For this review, take the finished solid that the model builds, in its own axes (mm). Round coordinates to 2 decimals unless told otherwise and drop trailing zeros. Loops run counter-clockwise (first coordinate to the right, second up) from the corner with the lowest first, then second, coordinate; pieces in that order, holes last. Notation, with made-up numbers: (43.5, -26.75) -> (80.5, -26.75) arc R18 cw to (80.5, -0.75) -> close; hole circle Ø11 at (84, 13). An arc over 180 degrees is marked (long way). One line per question, with ' | ' between items. Start each with the question number.
1. Draft analysis for pull direction Y (two halves, no side actions). For faces 1 (the face through (97, 79, 0)), 2 (the face through (46.24, 97.88, 1.48)), state which applies: pulls with the +Y half, pulls with the -Y half, needs draft (parallel to the pull), parting line crosses it, or undercut.
2. Wall thickness on line 1 along Y through (x, z) = (64.5, 2.1); line 2 along Y through (x, z) = (52.5, 1.65); line 3 along Y through (x, z) = (45.5, 2.45): over which ranges is each line inside the solid? List them lowest first.
3. Consider section A-A (y = 139.5). Write out the cut boundary in (x, z).
4. For pin 1 Ø5.5 at (x, y) = (95.5, 73.8) entering from +Z, flat-tipped, find the tip position at first contact; note if it passes through.
5. Consider section B-B (z = 1.55). Count the separate pieces of the cut face and the enclosed holes in it, and give its area (3 significant figures).
6. Consider section C-C (x = 27.5). Write out the cut boundary in (y, z), and give its area (3 significant figures).
```python
from build123d import *

# Parameters (mm, degrees)
MODEL_R                         = 3.59
MODEL_R_2                       = 2.55
MODEL_R_3                       = 1.7
MODEL_R_4                       = 2.7
AUFSATZ_LINEAR_AUSTRAGEN1_DEPTH = 3


with BuildPart() as part:
    # Model → Aufsatz-Linear austragen1 (new body)
    with BuildSketch(Plane.XY):
        with BuildLine():
            Line((157, 155), (47.6787101, 155))
            ThreePointArc((47.6787101, 155), (42.610842111, 153.620714242), (38.94098175, 149.86334281))
            Line((38.94098175, 149.86334281), (1.26227165, 82.167861266))
            ThreePointArc((1.26227165, 82.167861266), (0.32071068, 79.816760135), (0, 77.304518457))
            Line((0, 77.304518457), (0, 10))
            ThreePointArc((0, 10), (2.928932188, 2.928932188), (10, 0))
            Line((10, 0), (150, 0))
            ThreePointArc((150, 0), (157.071067812, 2.928932188), (160, 10))
            Line((160, 10), (160, 152))
            ThreePointArc((160, 152), (159.121320344, 154.121320344), (157, 155))
        make_face()
        with Locations((12.7, 12.7)):
            Circle(MODEL_R, mode=Mode.SUBTRACT)
        with Locations((47.7, 12.7)):
            Circle(MODEL_R, mode=Mode.SUBTRACT)
        with Locations((147.3, 12.7)):
            Circle(MODEL_R, mode=Mode.SUBTRACT)
        with Locations((47.7, 145)):
            Circle(MODEL_R, mode=Mode.SUBTRACT)
        with Locations((112.3, 145)):
            Circle(MODEL_R_2, mode=Mode.SUBTRACT)
        with Locations((52.5, 76.5)):
            Circle(MODEL_R_2, mode=Mode.SUBTRACT)
        with Locations((107.5, 76.5)):
            Circle(MODEL_R_2, mode=Mode.SUBTRACT)
        with Locations((64.5, 39)):
            Circle(MODEL_R_2, mode=Mode.SUBTRACT)
        with Locations((95.5, 39)):
            Circle(MODEL_R_2, mode=Mode.SUBTRACT)
        with Locations((64.5, 61.8)):
            Circle(MODEL_R_3, mode=Mode.SUBTRACT)
        with Locations((64.5, 73.8)):
            Circle(MODEL_R_3, mode=Mode.SUBTRACT)
        with Locations((64.5, 92.8)):
            Circle(MODEL_R_3, mode=Mode.SUBTRACT)
        with Locations((64.5, 104.8)):
            Circle(MODEL_R_3, mode=Mode.SUBTRACT)
        with Locations((95.5, 61.8)):
            Circle(MODEL_R_3, mode=Mode.SUBTRACT)
        with Locations((95.5, 73.8)):
            Circle(MODEL_R_3, mode=Mode.SUBTRACT)
        with Locations((95.5, 92.8)):
            Circle(MODEL_R_3, mode=Mode.SUBTRACT)
        with Locations((95.5, 104.8)):
            Circle(MODEL_R_3, mode=Mode.SUBTRACT)
        with Locations((56.38, 53.68)):
            Circle(MODEL_R_4, mode=Mode.SUBTRACT)
        with Locations((103.62, 53.68)):
            Circle(MODEL_R_4, mode=Mode.SUBTRACT)
        with Locations((103.62, 100.92)):
            Circle(MODEL_R_4, mode=Mode.SUBTRACT)
        with Locations((56.38, 100.92)):
            Circle(MODEL_R_4, mode=Mode.SUBTRACT)
        with Locations((70, 145)):
            Circle(MODEL_R_4, mode=Mode.SUBTRACT)
        with Locations((150, 145)):
            Circle(MODEL_R_4, mode=Mode.SUBTRACT)
        with Locations((150, 125)):
            Circle(MODEL_R_4, mode=Mode.SUBTRACT)
        with Locations((108.8, 139.5)):
            Circle(MODEL_R_2, mode=Mode.SUBTRACT)
        with Locations((80, 61.8)):
            Circle(MODEL_R_4, mode=Mode.SUBTRACT)
        with Locations((113.403724343, 95.203724343)):
            Circle(MODEL_R_4, mode=Mode.SUBTRACT)
        with Locations((80, 128.607448687)):
            Circle(MODEL_R_4, mode=Mode.SUBTRACT)
        with Locations((46.596275657, 95.203724343)):
            Circle(MODEL_R_4, mode=Mode.SUBTRACT)
        with Locations((90, 10)):
            Circle(MODEL_R_4, mode=Mode.SUBTRACT)
        with Locations((70, 10)):
            Circle(MODEL_R_4, mode=Mode.SUBTRACT)
        with Locations((69.999999708, 125.000000186)):
            Circle(MODEL_R_4, mode=Mode.SUBTRACT)
        with BuildLine():
            Line((68.75, 89.3), (68.75, 77.3))
            ThreePointArc((68.75, 77.3), (80, 66.05), (91.25, 77.3))
            Line((91.25, 77.3), (91.25, 89.3))
            ThreePointArc((91.25, 89.3), (80, 100.55), (68.75, 89.3))
        make_face(mode=Mode.SUBTRACT)
        with BuildLine():
            Line((130, 147.7), (125, 147.7))
            ThreePointArc((125, 147.7), (122.3, 145), (125, 142.3))
            Line((125, 142.3), (130, 142.3))
            ThreePointArc((130, 142.3), (132.7, 145), (130, 147.7))
        make_face(mode=Mode.SUBTRACT)
        with BuildLine():
            Line((129.999999456, 127.699999985), (124.999999456, 127.699999985))
            ThreePointArc((124.999999456, 127.699999985), (122.299999456, 124.999999985), (124.999999456, 122.299999985))
            Line((124.999999456, 122.299999985), (129.999999456, 122.299999985))
            ThreePointArc((129.999999456, 122.299999985), (132.699999456, 124.999999985), (129.999999456, 127.699999985))
        make_face(mode=Mode.SUBTRACT)
        with BuildLine():
            Line((99.999999456, 127.699999985), (89.999999456, 127.699999985))
            ThreePointArc((89.999999456, 127.699999985), (87.299999456, 124.999999985), (89.999999456, 122.299999985))
            Line((89.999999456, 122.299999985), (99.999999456, 122.299999985))
            ThreePointArc((99.999999456, 122.299999985), (102.699999456, 124.999999985), (99.999999456, 127.699999985))
        make_face(mode=Mode.SUBTRACT)
        with BuildLine():
            Line((99.999999587, 147.700000259), (89.999999587, 147.700000259))
            ThreePointArc((89.999999587, 147.700000259), (87.299999587, 145.000000259), (89.999999587, 142.300000259))
            Line((89.999999587, 142.300000259), (99.999999587, 142.300000259))
            ThreePointArc((99.999999587, 142.300000259), (102.699999587, 145.000000259), (99.999999587, 147.700000259))
        make_face(mode=Mode.SUBTRACT)
        with BuildLine():
            Line((5.5, 55.15), (3.5, 55.15))
            ThreePointArc((3.5, 55.15), (2.35, 54), (3.5, 52.85))
            Line((3.5, 52.85), (5.5, 52.85))
            ThreePointArc((5.5, 52.85), (6.65, 54), (5.5, 55.15))
        make_face(mode=Mode.SUBTRACT)
        with BuildLine():
            Line((5.5, 61.65), (3.5, 61.65))
            ThreePointArc((3.5, 61.65), (2.35, 60.5), (3.5, 59.35))
            Line((3.5, 59.35), (5.5, 59.35))
            ThreePointArc((5.5, 59.35), (6.65, 60.5), (5.5, 61.65))
        make_face(mode=Mode.SUBTRACT)
        with BuildLine():
            Line((156.5, 55.15), (154.5, 55.15))
            ThreePointArc((154.5, 55.15), (153.35, 54), (154.5, 52.85))
            Line((154.5, 52.85), (156.5, 52.85))
            ThreePointArc((156.5, 52.85), (157.65, 54), (156.5, 55.15))
        make_face(mode=Mode.SUBTRACT)
        with BuildLine():
            Line((156.5, 61.65), (154.5, 61.65))
            ThreePointArc((154.5, 61.65), (153.35, 60.5), (154.5, 59.35))
            Line((154.5, 59.35), (156.5, 59.35))
            ThreePointArc((156.5, 59.35), (157.65, 60.5), (156.5, 61.65))
        make_face(mode=Mode.SUBTRACT)
        with BuildLine():
            ThreePointArc((109.310874569, 12.798300857), (106.696941428, 8.857902693), (111.314549159, 9.876275414))
            ThreePointArc((111.314549159, 9.876275414), (111.482776901, 10.139700353), (111.789125431, 10.201699143))
            ThreePointArc((111.789125431, 10.201699143), (114.403058572, 14.142097307), (109.785450841, 13.123724586))
            ThreePointArc((109.785450841, 13.123724586), (109.617223099, 12.860299647), (109.310874569, 12.798300857))
        make_face(mode=Mode.SUBTRACT)
        with BuildLine():
            ThreePointArc((147.201699143, 74.310874569), (151.142097307, 71.696941428), (150.123724586, 76.314549159))
            ThreePointArc((150.123724586, 76.314549159), (149.860299647, 76.482776901), (149.798300857, 76.789125431))
            ThreePointArc((149.798300857, 76.789125431), (145.857902693, 79.403058572), (146.876275414, 74.785450841))
            ThreePointArc((146.876275414, 74.785450841), (147.139700353, 74.617223099), (147.201699143, 74.310874569))
        make_face(mode=Mode.SUBTRACT)
        with BuildLine():
            ThreePointArc((13.123724586, 74.785450841), (14.142097307, 79.403058572), (10.201699143, 76.789125431))
            ThreePointArc((10.201699143, 76.789125431), (10.139700353, 76.482776901), (9.876275414, 76.314549159))
            ThreePointArc((9.876275414, 76.314549159), (8.857902693, 71.696941428), (12.798300857, 74.310874569))
            ThreePointArc((12.798300857, 74.310874569), (12.860299647, 74.617223099), (13.123724586, 74.785450841))
        make_face(mode=Mode.SUBTRACT)
    extrude(amount=AUFSATZ_LINEAR_AUSTRAGEN1_DEPTH)


solid = part.part
```
Answer block:
1) face 1: needs draft | face 2: undercut
2) line 1: y = 0 to 36.45, 41.55 to 60.1, 63.5 to 72.1, 75.5 to 91.1, 94.5 to 103.1, 106.5 to 155 | line 2: y = 0 to 73.95, 79.05 to 155 | line 3: y = 0 to 9.86, 15.54 to 92.74, 97.67 to 142.16, 147.84 to 154.76
3) outline: (33.17, 0) -> (106.25, 0) -> (106.25, 3) -> (33.17, 3) -> close; (111.35, 0) -> (160, 0) -> (160, 3) -> (111.35, 3) -> close
4) pin 1: stops at z = 3
5) separate pieces: 1 | enclosed holes: 44 | area: 21,400 mm2
6) outline: (0, 0) -> (129.31, 0) -> (129.31, 3) -> (0, 3) -> close | area: 388 mm2
